Autodesk Inventor part; units mm, degrees
ref_plane "YZ Plane" through (0, 0, 0) normal (1, 0, 0) x (0, 1, 0)
ref_plane "XZ Plane" through (0, 0, 0) normal (0, 1, 0) x (-1, 0, 0)
ref_plane "XY Plane" through (0, 0, 0) normal (0, 0, 1) x (1, 0, 0)
sketch "Sketch1" plane through (0, 0, 0) normal (0, 1, 0) x (-1, 0, 0)
  line L0 (0, 0) -> (0, -1000)
  line L1 (0, -1000) -> (150, -1000)
  line L2 (150, -1000) -> (150, 0)
  circle A0 centre (150, 0) radius 150
  circle A1 centre (150, -1000) radius 150
  line L3 (300, 0) -> (300, -1000)
  circle A2 centre (150, 0) radius 75
  circle A3 centre (150, -1000) radius 75
  dimension "d0" = 1000
  dimension "d1" = 150
  dimension "d2" = 1000
  dimension "d3" = 150
  dimension "d4" = 150
extrude "Extrusion1" add sketch "Sketch1" along normal blind 300 contours A0 L2 A1 L0 | A0 | A1 L2 A3 L1 | L1 A3 L2 A1 | L3 A1 L2 A0
sketch "Sketch2" plane through (0, 0, 0) normal (0, -1, 0) x (1, 0, 0)
  line L0 (0, 0) -> (-300, 0)
  line L1 (0, 140) -> (-300, 140)
  circle A0 centre (-150, 0) radius 150
  circle A1 centre (-150, -1000) radius 75
  circle A2 centre (-150, -1000) radius 150
  arc A3 (-300, -1000) -> (0, -1000) centre (-150, -1000) ccw
  line L2 (-300, -1000) -> (0, -1000)
  line L3 (-300, -1140) -> (0, -1140)
  point P0 (-96.1484, -1140)
  point P1 (-203.8516, -1140)
  point P2 (-203.8516, 140)
  point P3 (-96.1484, 140)
  dimension "d7" = 140
  dimension "d8" = 140
extrude "Extrusion2" cut sketch "Sketch2" against normal through all contours L1 A0 | A2 L3
equation "\"BendRadius\" = Thickness"
equation "\"BendReliefWidth\" = Thickness"
equation "\"BendReliefDepth\" = 0.5 * Thickness"
equation "\"CornerReliefSize\" = 4 * Thickness"
equation "\"MinimumRemnant\" = 2 * Thickness"
equation "\"TransitionRadius\" = BendRadius"
equation "\"JacobiRadiusSize\" = BendRadius"
equation "\"GapSize\" = Thickness"
properties part number "Middle v2" material "Steel"
Can you work these out from the model? Positions are in its coordinate system, mm. Coordinates: 2 decimals unless noted, no trailing zeros. Loops run counter-clockwise (first coordinate to the right, second up) from the corner with the lowest first, then second, coordinate; pieces in that order, holes last. Notation, with made-up numbers: M -22,-35.5 L 35,-35.5 A9 cw 35,-26.5 Z; hole C 75,41.5 d11. An arc over 180 degrees is marked long. Answer as CSV lines item,"result". Start each with the question number.
1. If I drill on probe 1 along Z at (x, y) = (-150, 187); probe 2 along Z at (x, y) = (-146.5, 34); probe 3 along X at (y, z) = (142, -1000), over which ranges is the centre line in solid material (lowest first)? Write a range as [from, to].
2. Suppose I cut it at D-D, the plane x = -269. List the corners of the cut face in (y, z) for me.
3. Thinking about a two-plate mould opening in X: for faces 1 (the face through (-148, 0, -491)), 2 (the face through (0, 148, -493)), 3 (the face through (-221.537, 147.9, -22.528)), which applies, +X half, -X half, draft (parallel to the pull), parting line (faces both ways), or undercut?
4. Suppose I cut it at B-B, the plane y = 231. List the corners of the cut face in (x, z) for me.
5. Suppose I cut it at A-A, the plane x = -129. List the corners of the cut face in (y, z) for me, plus the area to 3 significant figures.
6. Suppose I cut it at C-C, the plane x = -33. List the corners of the cut face in (y, z) for me, plus the area to 3 significant figures.
Output:
1,probe 1,"z = [-1140, -1075], [-925, -75], [75, 140]"
1,probe 2,"z = [-1140, -1074.92], [-925.08, -74.92], [74.92, 140]"
1,probe 3,"x = [-300, -225], [-75, 0]"
2,outline,"M 0,-1091.32 L 300,-1091.32 L 300,91.32 L 0,91.32 Z"
3,face 1,"draft"
3,face 2,"+X half"
3,face 3,"undercut"
4,outline,"M -300,-1000 A150 ccw -203.85,-1140 L -96.15,-1140 A150 ccw 0,-1000 L 0,0 A150 ccw -96.15,140 L -203.85,140 A150 ccw -300,0 Z; hole C -150,-1000 d150; hole C -150,0 d150"
5,outline,"M 0,-1140 L 300,-1140 L 300,-1072 L 0,-1072 Z; M 0,-928 L 300,-928 L 300,-72 L 0,-72 Z; M 0,72 L 300,72 L 300,140 L 0,140 Z"
5,area,"298,000 mm^2"
6,outline,"M 0,-1093.87 L 300,-1093.87 L 300,93.87 L 0,93.87 Z"
6,area,"356,000 mm^2"
